Can you work these out from the drawing? Everything is in mm from the part's minimum corner. A direction names the side the tool comes from. Give positions to 0.01 mm unless a question says otherwise; leave off trailing zeros. Write each loop counter-clockwise with the first axis right and the second up, starting at its lowest first coordinate (ties: lowest second). Pieces come first, ordered by that corner, then holes. Notation, with made-up numbers: (-21, 77) -> (21, 77) arc R26 cw to (21, 100) -> close; hole circle Ø1 at (76, 25). An arc over 180 degrees is marked (long way). Return JSON: item names as keys, results as strings.
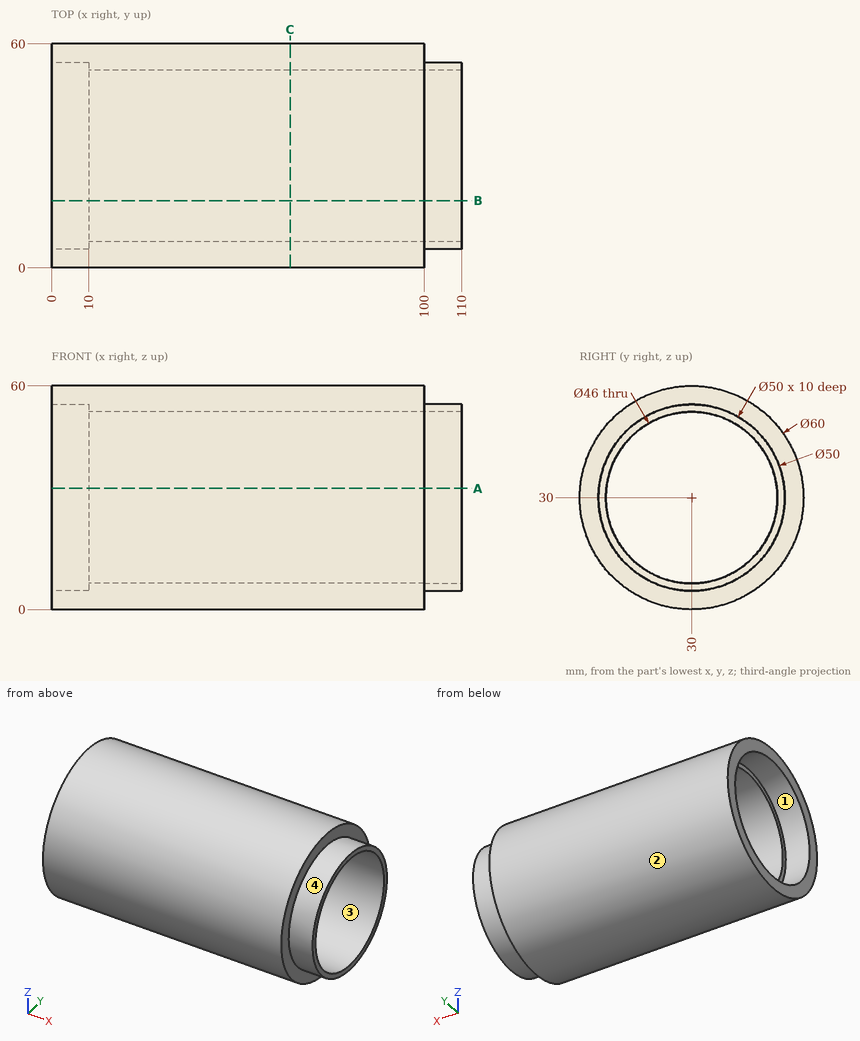
1. If I drill on line 1 (Y direction, x = 80.5, z = 30); line 2 (X direction, y = 39, z = 8); line 3 (Y direction, x = 25.5, z = 25), over which ranges is the centre line in solid material (lowest first)? Write a range as [from, to].
Taken from the geometry:
{"line 1": "y = [0, 7], [53, 60]", "line 2": "x = [10, 110]", "line 3": "y = [0.42, 7.55], [52.45, 59.58]"}
2. Suppose I cut it at B-B, the plane y = 18. List the corners of the cut face in (x, z) for me, and give its area (3 significant figures).
Taken from the geometry:
{"outline": "(0, 2.5) -> (100, 2.5) -> (100, 8.07) -> (110, 8.07) -> (110, 10.38) -> (10, 10.38) -> (10, 8.07) -> (0, 8.07) -> close; (0, 51.93) -> (10, 51.93) -> (10, 49.62) -> (110, 49.62) -> (110, 51.93) -> (100, 51.93) -> (100, 57.5) -> (0, 57.5) -> close", "area": "1,570 mm²"}
3. For pin 1 Ø5 at (x, z) = (95, 23) entering from -Y; pin 2 Ø6 at (x, y) = (50, 29.5) entering from +Z; pin 3 Ø2 at (x, y) = (18, 44) entering from -Z, each with a flat end and sliding along its axis, tell me the tip position at first contact or that it passes through.
Taken from the geometry:
{"pin 1": "stops at y = 0.34", "pin 2": "stops at z = 60", "pin 3": "stops at z = 2.96"}
4. Suppose I cut it at C-C, the plane x = 64. List the corners of the cut face in (y, z) for me, and give its area (3 significant figures).
Taken from the geometry:
{"outline": "circle Ø60 at (30, 30); hole circle Ø46 at (30, 30)", "area": "1,170 mm²"}
5. Suppose I cut it at A-A, the plane z = 32.5. List the corners of the cut face in (x, y) for me, and give its area (3 significant figures).
Taken from the geometry:
{"outline": "(0, 0.1) -> (100, 0.1) -> (100, 5.13) -> (110, 5.13) -> (110, 7.14) -> (10, 7.14) -> (10, 5.13) -> (0, 5.13) -> close; (0, 54.87) -> (10, 54.87) -> (10, 52.86) -> (110, 52.86) -> (110, 54.87) -> (100, 54.87) -> (100, 59.9) -> (0, 59.9) -> close", "area": "1,410 mm²"}
6. If we mould it in two halves opening along Y, with no side actions, what happens to the marked faces 1 and 2? For each: released by +Y, released by -Y, zero draft, split by the parting line, or undercut.
Taken from the geometry:
{"face 1": "undercut", "face 2": "split by the parting line"}
7. Which directions (+Z, -Z, +X, -X, +Y, -Y) give clear straight access to the entire face, cutting with the end or side of a thin tool? Please do the marked faces 3 and 4.
Taken from the geometry:
{"face 3": "+X, -X", "face 4": "+X"}
